The listing builds one solid part. Answer for the finished solid, in the listing's coordinates (mm). Face numbers are marked on the shaded views. A direction names the side the tool comes from. Give positions to 0.01 mm unless a question says otherwise; leave off trailing zeros. Order: outer loops, then holes, each group sorted by start corner. A loop starts at its lowest first (then second) coordinate and runs counter-clockwise, first axis right, second up.
```python
from build123d import *

# Parameters (mm, degrees)
F0_W     = 58
F0_H     = 20
F0_R     = 2
F1_DEPTH = 2.54
F2_W     = 32.392131
F2_H     = 20
F3_DEPTH = 25.4
F4_W     = 20
F4_H     = 2.54
F5_DEPTH = 46
F6_W     = 55
F6_H     = 0.7
F7_DEPTH = 20.001


with BuildPart() as f1:
    # F0 (on Top) → F1 (new body)
    with BuildSketch(Plane.XY):
        Rectangle(F0_W, F0_H)
        with Locations((-25, -5)):
            Circle(F0_R, mode=Mode.SUBTRACT)
        with Locations((25, -5)):
            Circle(F0_R, mode=Mode.SUBTRACT)
        with Locations((-25, 5)):
            Circle(F0_R, mode=Mode.SUBTRACT)
        with Locations((25, 5)):
            Circle(F0_R, mode=Mode.SUBTRACT)
    extrude(amount=F1_DEPTH)

    # F2 (on face) → F3 (join)
    with BuildSketch(Plane.XY.offset(2.54)):
        with Locations((0.897951, 0)):
            Rectangle(F2_W, F2_H)
    extrude(amount=F3_DEPTH)

    # F4 (on face) → F5 (join)
    with BuildSketch(Plane.YZ.offset(17.094016)):
        with Locations((0, 26.67)):
            Rectangle(F4_W, F4_H)
    extrude(amount=F5_DEPTH)

    # F6 (on face) → F7 (cut, through all)
    with BuildSketch(Plane(origin=(0, 10, 0), x_dir=(-1, 0, 0), z_dir=(0, 1, 0))):
        with Locations((-30.594016, 26.701)):
            Rectangle(F6_W, F6_H)
    extrude(amount=-F7_DEPTH, mode=Mode.SUBTRACT)


solid = f1.part
```
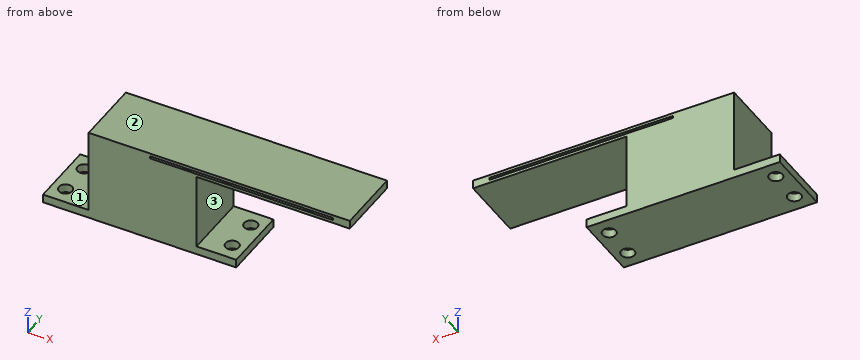
1) Find section A-A (x = 25). Write down the section's boundary in (y, z), then the cut area to 3 significant figures.
Geometry says:
outline: (-10, 0) - (-7, 0) - (-7, 2.54) - (-10, 2.54) - close; (-10, 25.4) - (10, 25.4) - (10, 26.35) - (-10, 26.35) - close; (-10, 27.05) - (10, 27.05) - (10, 27.94) - (-10, 27.94) - close; (-3, 0) - (3, 0) - (3, 2.54) - (-3, 2.54) - close; (7, 0) - (10, 0) - (10, 2.54) - (7, 2.54) - close
area: 67.3 mm2
2) Find section D-D (z = 8.75). Write down the section's boundary in (x, y), then the cut area to 3 significant figures.
Geometry says:
outline: (-15.3, -10) - (17.09, -10) - (17.09, 10) - (-15.3, 10) - close
area: 648 mm2
3) Find section C-C (x = -25). Write down the section's boundary in (y, z).
Geometry says:
outline: (-10, 0) - (-7, 0) - (-7, 2.54) - (-10, 2.54) - close; (-3, 0) - (3, 0) - (3, 2.54) - (-3, 2.54) - close; (7, 0) - (10, 0) - (10, 2.54) - (7, 2.54) - close
4) Find section B-B (y = -5). Write down the section's boundary in (x, z), then the cut area to 3 significant figures.
Geometry says:
outline: (-29, 0) - (-27, 0) - (-27, 2.54) - (-29, 2.54) - close; (-23, 0) - (23, 0) - (23, 2.54) - (17.09, 2.54) - (17.09, 25.4) - (63.09, 25.4) - (63.09, 27.94) - (-15.3, 27.94) - (-15.3, 2.54) - (-23, 2.54) - close; (27, 0) - (29, 0) - (29, 2.54) - (27, 2.54) - close; hole (3.09, 26.35) - (58.09, 26.35) - (58.09, 27.05) - (3.09, 27.05) - close
area: 1,030 mm2
5) A tool of negligible diameter and unlimited length cuts with its end or side. For the marked faces 1, 2 and 3, from which of +Z, -Z, +X, -X, +Y, -Y can it reach the whole face along a straight path? Write none if from no direction.
Geometry says:
face 1: +Z, -X, +Y, -Y
face 2: +Z, +X, -X, +Y, -Y
face 3: +X, +Y, -Y
6) Straight lines are drawn through the part: probe 1 along Y at (x, z) = (25, 2.05); probe 2 along Z at (x, y) = (20.5, 3.75); probe 3 along Z at (x, y) = (40.5, -3). For each, find the intervals that lie inside material, in ascending order.
Geometry says:
probe 1: y = -10 to -7, -3 to 3, 7 to 10
probe 2: z = 0 to 2.54, 25.4 to 26.35, 27.05 to 27.94
probe 3: z = 25.4 to 26.35, 27.05 to 27.94
7) Given P1, Ø0.8, axis at y = 0, z = 26.5, coming from the -X side; P2, Ø2, axis at y = -4.5, z = 2, coming from the +X side; P3, Ø3.5, axis at x = 25, y = 5, coming from the -Z side, each flat-ended and moving along its own axis, determine where each tip first touches the part or whether it passes through.
Geometry says:
P1: stops at x = -15.3
P2: stops at x = 29
P3: stops at z = 25.4
